For this review, use the dimensioned drawing (mm, ordinates from the lowest corner) and the shaded views. A direction names the side the tool comes from. Coordinates: 2 decimals unless noted, no trailing zeros. Loops run counter-clockwise (first coordinate to the right, second up) from the corner with the lowest first, then second, coordinate; pieces in that order, holes last. Notation, with made-up numbers: (69, 22.5) - (109, 22.5) arc R16 ccw to (109, 43.5) - close; hole circle Ø7 at (47.25, 27). An arc over 180 degrees is marked (long way). Use a Markdown table: item, result. Add a question column.
1) To check wall thickness, follow L1, parallel to Y at x = 2.9, z = 28; L2, parallel to Z at x = 0.75, y = 6.5; L3, parallel to Z at x = 1.5, y = 4.75. State the ranges of each line that lie inside material, in increasing order. Write a range as [from, to].
2) The part is to be moulded in two halves that separate along Z. For the marked faces 4, 5 and 6, say which applies: pulls with the +Z half, pulls with the -Z half, needs draft (parallel to the pull), parting line crosses it, or undercut.
3) Clearance check with flat-ended pins moving along their axes: pin 1 (1 mm diameter, centred on x = 2.5, y = 14, fed in from +Z); pin 2 (1 mm diameter, centred on x = 1.5, z = 6.5, fed in from -Y); pin 3 (1.6 mm diameter, centred on x = 1.5, z = 7.5, fed in from +Y). State where each tip first meets the part, or that it passes through.
4) Add section C-C, the plane z = 30.5. Give the boundary of the cut face in (x, y) (1 decimal).
5) For the marked faces 1, 2 and 3, list the 3-axis set-ups (+Z, -Z, +X, -X, +Y, -Y) from which the entire face can be reached by the end or side of a thin tool; tool diameter is ignored.
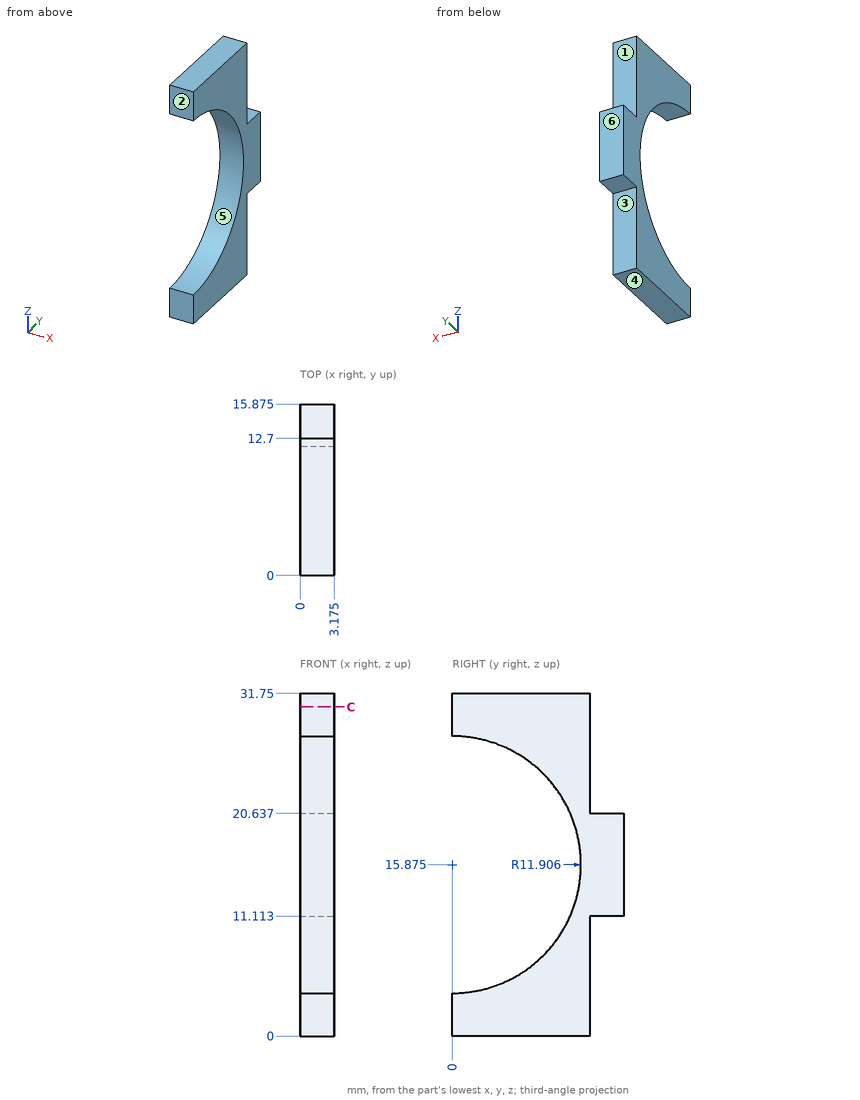
From the geometry:
| question | item | result |
|---|---|---|
| 1 | L1 | y = [0, 12.7] |
| 1 | L2 | z = [0, 5.9], [25.85, 31.75] |
| 1 | L3 | z = [0, 4.96], [26.79, 31.75] |
| 2 | face 4 | pulls with the -Z half |
| 2 | face 5 | undercut |
| 2 | face 6 | needs draft |
| 3 | pin 1 | stops at z = 20.64 |
| 3 | pin 2 | stops at y = 6.65 |
| 3 | pin 3 | stops at y = 12.7 |
| 4 | outline | (0, 0) - (3.2, 0) - (3.2, 12.7) - (0, 12.7) - close |
| 5 | face 1 | +Z, +X, -X, +Y |
| 5 | face 2 | +Z, -Z, +X, -X, -Y |
| 5 | face 3 | -Z, +X, -X, +Y |
